Could you check a few things on this model? Use its own coordinates, in mm. A direction names the side the tool comes from. Give positions to 0.01 mm unless a question says otherwise; leave off trailing zeros. Loops run counter-clockwise (first coordinate to the right, second up) from the corner with the lowest first, then second, coordinate; pieces in that order, holes last. Notation, with made-up numbers: (64.5, -35.5) -> (108.5, -35.5) arc R25 cw to (108.5, -1.5) -> close; hole circle Ø1 at (37.25, -1). An arc over 180 degrees is marked (long way). Write item = value, one per line. Start each with the question number.
1) I need wall thicknesses on probe 1 along Z at (x, y) = (6.75, 2.25); probe 2 along Y at (x, z) = (1.5, 3); probe 3 along X at (y, z) = (12, 21.5) (3 decimals). Which ranges of each line are inside material? Lowest first, please. Write a range as from..to.
2) I'm going to push flat-ended pins straight in: pin 1 Ø3.5 at (x, z) = (5, 6) entering from +Y; pin 2 Ø5 at (x, y) = (11, 5) entering from +Z; pin 3 Ø5 at (x, z) = (9.5, 11.5) entering from +Y; pin 4 Ø1 at (y, z) = (8, 11) entering from +X. Where does each tip first touch, or does it pass through?
3) If we mould it in two halves opening along X, with no side actions, what happens to faces 3 (the face through (6.67, 9.09, 23.92)), 4 (the face through (0.905, 13.96, 26.19)), 5 (the face through (8.04, 0.25, 18.97))? For each: +X half, -X half, draft (parallel to the pull), parting line (faces both ways), or undercut.
4) I want a section at A-A (z = 7). List the corners of the cut face in (x, y) for me (3 decimals).
5) On a 3-axis mill with a long thin cutter (end or side, diameter ignored), from which of +Z, -Z, +X, -X, +Y, -Y can I reach the whole of each face in a straight line? I mean faces 1 (the face through (8, 6.35, 6)), 2 (the face through (8, 0, 9)). Say none if no direction works.
from build123d import *

# Parameters (mm, degrees)
BOSS_EXTRUDE1_DEPTH = 15.875
SKETCH2_R           = 3.302
CUT_EXTRUDE1_DEPTH  = 38.921561078
CHAMFER1_SIZE       = 3.175
CHAMFER1_SIZE2      = 3.652419693
FILLET1_R           = 3.175
FILLET2_R           = 0.508


with BuildPart() as part:
    # Sketch1 → Boss-Extrude1 (new body)
    with BuildSketch(Plane(origin=(0, 0, 0), x_dir=(0, 0, -1), z_dir=(1, 0, 0))):
        Polygon((0, 0), (-19.05, 0), (-30.275320151, 11.225320151), (-23.540128061, 17.960512242), (-11.929615818, 6.35), (0, 6.35), align=None)
    extrude(amount=BOSS_EXTRUDE1_DEPTH)

    # Sketch2 → Cut-Extrude1 (cut, through all)
    with BuildSketch(Plane(origin=(0, -2.789807909, 2.789807909), x_dir=(1, 0, 0), z_dir=(0, 0.7071067811865465, -0.7071067811865486))):
        with Locations(Location((7.9375, -20.291640303, 0), (0, 0, 270))):
            Circle(SKETCH2_R)
    extrude(amount=-CUT_EXTRUDE1_DEPTH, mode=Mode.SUBTRACT)

    # Chamfer1
    chamfer1_edges = [part.edges().sort_by_distance(p)[0] for p in [
        (7.9375, 9.223681959, 14.803297777),
    ]]
    chamfer1_side = [part.faces().sort_by_distance(p)[0] for p in [
        (7.9375, 17.799015553, 23.378631371),
    ]]
    chamfer(chamfer1_edges, length=CHAMFER1_SIZE, length2=CHAMFER1_SIZE2, reference=chamfer1_side[0])

    # Fillet1
    fillet1_edges = [part.edges().sort_by_distance(p)[0] for p in [
        (7.9375, 0, 19.05),
        (15.875, 14.592916197, 26.907724106),
        (15.875, 3.175, 0),
        (0, 14.592916197, 26.907724106),
        (0, 3.175, 0),
    ]]
    fillet(fillet1_edges, radius=FILLET1_R)

    # Fillet2
    fillet2_edges = [part.edges().sort_by_distance(p)[0] for p in [
        (7.9375, 6.35, 11.929615818),
        (15.875, 11.032724106, 16.612339924),
        (7.9375, 6.35, 0),
        (7.9375, 0, 0),
        (0, 6.35, 7.552307909),
        (15.875, 6.35, 7.552307909),
        (14.94506403, 6.35, 0.92993597),
        (0.92993597, 6.35, 0.92993597),
        (0, 0, 10.45493597),
        (0, 4.955096045, 24.005096045),
        (0, 0.241682484, 18.949891837),
        (15.875, 0, 10.45493597),
        (14.94506403, 0, 0.92993597),
        (0.92993597, 0, 0.92993597),
        (15.875, 4.955096045, 24.005096045),
        (15.875, 0.241682484, 18.949891837),
        (7.9375, 11.225320151, 30.275320151),
        (7.9375, 17.960512242, 23.540128061),
        (14.94506403, 10.567756121, 29.617756121),
        (0.92993597, 10.567756121, 29.617756121),
        (14.94506403, 17.302948212, 22.88256403),
        (0.92993597, 17.302948212, 22.88256403),
        (0, 11.032724106, 16.612339924),
    ]]
    fillet(fillet2_edges, radius=FILLET2_R)


solid = part.part
Answer list:
q1.probe_1 = 0..21.3
q1.probe_2 = 0..6.35
q1.probe_3 = 0..5.7, 10.175..15.875
q2.pin_1 = 6.35
q2.pin_2 = 26.55
q2.pin_3 = 7.65
q2.pin_4 = through
q3.face_3 = undercut
q3.face_4 = -X half
q3.face_5 = draft
q4.outline = (0, 0.508) arc R0.508 ccw to (0.508, 0) -> (15.367, 0) arc R0.508 ccw to (15.875, 0.508) -> (15.875, 5.842) arc R0.508 ccw to (15.367, 6.35) -> (0.508, 6.35) arc R0.508 ccw to (0, 5.842) -> close
q5.face_1 = -Z, +X, -X, +Y
q5.face_2 = +Z, -Z, +X, -X, -Y
